Geometry: final body of the model. Coordinates: model frame, mm. A direction names the side the tool comes from. Give positions to 0.01 mm unless a question says otherwise; leave off trailing zeros. Write each loop counter-clockwise with the first axis right and the second up, starting at its lowest first coordinate (ties: lowest second). Pieces come first, ordered by that corner, then holes.
```python
from build123d import *

# Parameters (mm, degrees)
CROQUIS1_W              = 800
CROQUIS1_H              = 630
SALIENTE_EXTRUIR1_DEPTH = 10
SALIENTE_EXTRUIR3_DEPTH = 20
SALIENTE_EXTRUIR4_DEPTH = 10
CROQUIS5_R              = 12.5
SALIENTE_EXTRUIR5_DEPTH = 40
SALIENTE_EXTRUIR6_DEPTH = 20
CROQUIS7_W              = 20
CROQUIS7_H              = 152.276428112
SALIENTE_EXTRUIR7_DEPTH = 60
CORTAR_EXTRUIR1_DEPTH   = 140
CROQUIS9_R              = 12.5
SALIENTE_EXTRUIR8_DEPTH = 111


with BuildPart() as part:
    # Croquis1 → Saliente-Extruir1 (new body)
    with BuildSketch(Plane(origin=(0, 0, 0), x_dir=(1, 0, 0), z_dir=(0, 1, 0))):
        Rectangle(CROQUIS1_W, CROQUIS1_H)
    extrude(amount=SALIENTE_EXTRUIR1_DEPTH)

    # Croquis2 → Saliente-Extruir3 (add)
    with BuildSketch(Plane(origin=(400, 0, 0), x_dir=(0, 0, -1), z_dir=(1, 0, 0))):
        with BuildLine():
            Line((-33.293773854, 70), (33.293773854, 70))
            ThreePointArc((33.293773854, 70), (50.501066944, 64.574561329), (61.484552477, 50.2606043))
            Line((61.484552477, 50.2606043), (76.138214056, 10))
            Line((76.138214056, 10), (-76.138214056, 10))
            Line((-76.138214056, 10), (-61.484552477, 50.2606043))
            ThreePointArc((-61.484552477, 50.2606043), (-50.501066944, 64.574561329), (-33.293773854, 70))
        make_face()
    saliente_extruir3 = extrude(amount=-SALIENTE_EXTRUIR3_DEPTH)

    # Croquis4 → Saliente-Extruir4 (add)
    with BuildSketch(Plane(origin=(400, 0, 0), x_dir=(0, 0, -1), z_dir=(1, 0, 0))):
        Polygon((-33.293773854, 54.43375673), (-45.793773854, 47.216878365), (-45.793773854, 32.783121635), (-33.293773854, 25.56624327), (-20.793773854, 32.783121635), (-20.793773854, 47.216878365), align=None)
        Polygon((33.293773854, 54.43375673), (20.793773854, 47.216878365), (20.793773854, 32.783121635), (33.293773854, 25.56624327), (45.793773854, 32.783121635), (45.793773854, 47.216878365), align=None)
    saliente_extruir4 = extrude(amount=SALIENTE_EXTRUIR4_DEPTH)

    # Simetr_a1: Saliente-Extruir3, Saliente-Extruir4 across plane
    add(saliente_extruir3.mirror(Plane(origin=(0, 0, 0), x_dir=(0, 0, 1), z_dir=(1, 0, 0))))
    add(saliente_extruir4.mirror(Plane(origin=(0, 0, 0), x_dir=(0, 0, 1), z_dir=(1, 0, 0))))

    # Croquis5 → Saliente-Extruir5 (add)
    with BuildSketch(Plane(origin=(-380, 0, 0), x_dir=(0, 0, -1), z_dir=(1, 0, 0))):
        with Locations((-33.293773854, 40)):
            Circle(CROQUIS5_R)
        with Locations(Location((33.293773854, 40, 0), (0, 0, 180))):
            Circle(CROQUIS5_R)
    saliente_extruir5 = extrude(amount=SALIENTE_EXTRUIR5_DEPTH)

    # Croquis6 → Saliente-Extruir6 (add)
    with BuildSketch(Plane(origin=(-340, 0, 0), x_dir=(0, 0, -1), z_dir=(1, 0, 0))):
        with BuildLine():
            Line((-76.138214056, 10), (76.138214056, 10))
            Line((76.138214056, 10), (61.484552477, 50.2606043))
            ThreePointArc((61.484552477, 50.2606043), (50.501066944, 64.574561329), (33.293773854, 70))
            Line((33.293773854, 70), (-33.293773854, 70))
            ThreePointArc((-33.293773854, 70), (-50.501066944, 64.574561329), (-61.484552477, 50.2606043))
            Line((-61.484552477, 50.2606043), (-76.138214056, 10))
        make_face()
    saliente_extruir6 = extrude(amount=SALIENTE_EXTRUIR6_DEPTH)

    # Simetr_a2: Saliente-Extruir5, Saliente-Extruir6 across plane
    add(saliente_extruir5.mirror(Plane(origin=(0, 0, 0), x_dir=(0, 0, 1), z_dir=(1, 0, 0))))
    add(saliente_extruir6.mirror(Plane(origin=(0, 0, 0), x_dir=(0, 0, 1), z_dir=(1, 0, 0))))

    # Croquis7 → Saliente-Extruir7 (add)
    with BuildSketch(Plane(origin=(0, 10, 0), x_dir=(1, 0, 0), z_dir=(0, 1, 0))):
        with Locations((-55, 0)):
            Rectangle(CROQUIS7_W, CROQUIS7_H)
        with Locations((55, 0)):
            Rectangle(CROQUIS7_W, CROQUIS7_H)
    extrude(amount=SALIENTE_EXTRUIR7_DEPTH)

    # Croquis8 → Cortar-Extruir1 (cut)
    with BuildSketch(Plane(origin=(65, 0, 0), x_dir=(0, 0, -1), z_dir=(1, 0, 0))):
        with BuildLine():
            Line((61.484552477, 50.2606043), (76.138214056, 10))
            Line((76.138214056, 10), (76.138214056, 70))
            Line((76.138214056, 70), (33.293773854, 70))
            ThreePointArc((33.293773854, 70), (50.501066944, 64.574561329), (61.484552477, 50.2606043))
        make_face()
        with BuildLine():
            ThreePointArc((-61.484552477, 50.2606043), (-50.501066944, 64.574561329), (-33.293773854, 70))
            Line((-33.293773854, 70), (-76.138214056, 70))
            Line((-76.138214056, 70), (-76.138214056, 10))
            Line((-76.138214056, 10), (-61.484552477, 50.2606043))
        make_face()
    extrude(amount=-CORTAR_EXTRUIR1_DEPTH, mode=Mode.SUBTRACT)

    # Croquis9 → Saliente-Extruir8 (add)
    with BuildSketch(Plane(origin=(65, 0, 0), x_dir=(0, 0, -1), z_dir=(1, 0, 0))):
        with Locations(Location((33.293773854, 40, 0), (0, 0, 180))):
            Circle(CROQUIS9_R)
        with Locations((-33.293773854, 40)):
            Circle(CROQUIS9_R)
    extrude(amount=-SALIENTE_EXTRUIR8_DEPTH)


solid = part.part
```
Item 1: Reachability of faces 5 (the face through (65, 40, -1)), 6 (the face through (360.28, 32.39, 43.21)), 7 (the face through (-54.86, 64.427, 50.711)) from +Z, -Z, +X, -X, +Y, -Y: full face, straight path, thin tool, end or side. Return the list, or none.
Found:
face 5: +Z, -Z, +Y
face 6: none
face 7: +Z, +X, -X, +Y
Item 2: Section B-B, the plane z = 11.5. Return the cut outline in (x, y), plus the area to 3 significant figures.
Found:
outline: (-400, 0) - (400, 0) - (400, 70) - (380, 70) - (380, 10) - (340, 10) - (340, 70) - (320, 70) - (320, 10) - (65, 10) - (65, 70) - (45, 70) - (45, 10) - (-45, 10) - (-45, 70) - (-65, 70) - (-65, 10) - (-320, 10) - (-320, 70) - (-340, 70) - (-340, 10) - (-380, 10) - (-380, 70) - (-400, 70) - close
area: 15,200 mm2
Item 3: Section C-C, the plane x = -110.5. Return the cut outline in (y, z).
Found:
outline: (0, -315) - (10, -315) - (10, 315) - (0, 315) - close
Item 4: Line query: L1, parallel to X at y = 42, z = 20; L2, parallel to Y at x = -339, z = 111; L3, parallel to X at y = 9, z = -161. Output: solid intervals per line, ascending.
Found:
L1: x = -400 to -380, -340 to -320, -65 to -45, 45 to 65, 320 to 340, 380 to 400
L2: y = 0 to 10
L3: x = -400 to 400
Item 5: Pull-direction query (Z, two-part tool) for faces 1 (the face through (-360.28, 47.61, -43.21)), 2 (the face through (-54.86, 64.72, -50.29)), 3 (the face through (390, 70, 0)), 4 (the face through (390.14, 29.848, 68.914)); classes: +Z half, -Z half, draft (parallel to the pull), parting line (faces both ways), or undercut.
Found:
face 1: undercut
face 2: -Z half
face 3: draft
face 4: +Z half
Item 6: Section A-A, the plane x = -21. Return the cut outline in (y, z), plus the area to 3 significant figures.
Found:
outline: (0, -315) - (10, -315) - (10, 315) - (0, 315) - close; circle Ø25 at (40, -33.29); circle Ø25 at (40, 33.29)
area: 7,280 mm2
Item 7: Pin query (flat end, axial travel): pin 1 Ø1.5 at (y, z) = (55, -61) entering from +X (1 decimal); pin 2 Ø8 at (x, y) = (-405.5, 40) entering from -Z; pin 3 Ø3 at (x, z) = (173.5, 3.5) entering from +Y; pin 4 Ø11 at (x, y) = (-405, 41.5) entering from +Z. Return the tip coordinate at first contact, or that it passes through.
Found:
pin 1: passes through
pin 2: stops at z = -45.79
pin 3: stops at y = 10
pin 4: stops at z = 65.51
Item 8: Section D-D, the plane z = -187.5. Return the cut outline in (x, y), plus the area to 3 significant figures.
Found:
outline: (-400, 0) - (400, 0) - (400, 10) - (-400, 10) - close
area: 8,000 mm2
